from build123d import *

# Parameters (mm, degrees)
F0_R     = 2.5
F0_R_2   = 3.5
F0_W     = 15
F0_H     = 3
F1_DEPTH = 3


with BuildPart() as f1:
    # F0 (on Front) → F1 (new body)
    with BuildSketch(Plane.XZ):
        Polygon((107.5, -32.625), (115, -32.625), (115, 32.625), (107.5, 32.625), (92.5, 32.625), (57.5, 32.625), (42.5, 32.625), (7.5, 32.625), (-7.5, 32.625), (-42.5, 32.625), (-57.5, 32.625), (-92.5, 32.625), (-107.5, 32.625), (-115, 32.625), (-115, -32.625), (-107.5, -32.625), (-92.5, -32.625), (-57.5, -32.625), (-42.5, -32.625), (-7.5, -32.625), (7.5, -32.625), (42.5, -32.625), (57.5, -32.625), (92.5, -32.625), align=None)
        with Locations((-75, -22.375)):
            Circle(F0_R, mode=Mode.SUBTRACT)
        with Locations((-65, -22.375)):
            Circle(F0_R, mode=Mode.SUBTRACT)
        with Locations((-55, -22.375)):
            Circle(F0_R, mode=Mode.SUBTRACT)
        with Locations((-45, -22.375)):
            Circle(F0_R, mode=Mode.SUBTRACT)
        with Locations((-95, -12.375)):
            Circle(F0_R, mode=Mode.SUBTRACT)
        with Locations((-85, -12.375)):
            Circle(F0_R, mode=Mode.SUBTRACT)
        with Locations((-65, -12.375)):
            Circle(F0_R, mode=Mode.SUBTRACT)
        with Locations((-105, -2.375)):
            Circle(F0_R, mode=Mode.SUBTRACT)
        with Locations((-95, -2.375)):
            Circle(F0_R, mode=Mode.SUBTRACT)
        with BuildLine():
            Line((-55.5, -9.875), (-55, -9.875))
            Line((-55, -9.875), (-45, -9.875))
            Line((-45, -9.875), (-35, -9.875))
            Line((-35, -9.875), (-25, -9.875))
            Line((-25, -9.875), (-15, -9.875))
            Line((-15, -9.875), (-5, -9.875))
            Line((-5, -9.875), (-4.5, -9.875))
            ThreePointArc((-4.5, -9.875), (-3.085786, -10.460786), (-2.5, -11.875))
            Line((-2.5, -11.875), (-2.5, -12.375))
            Line((-2.5, -12.375), (-2.5, -12.875))
            ThreePointArc((-2.5, -12.875), (-3.085786, -14.289214), (-4.5, -14.875))
            Line((-4.5, -14.875), (-5, -14.875))
            Line((-5, -14.875), (-15, -14.875))
            Line((-15, -14.875), (-25, -14.875))
            Line((-25, -14.875), (-35, -14.875))
            Line((-35, -14.875), (-45, -14.875))
            Line((-45, -14.875), (-55, -14.875))
            Line((-55, -14.875), (-55.5, -14.875))
            ThreePointArc((-55.5, -14.875), (-56.914214, -14.289214), (-57.5, -12.875))
            Line((-57.5, -12.875), (-57.5, -12.375))
            Line((-57.5, -12.375), (-57.5, -11.875))
            ThreePointArc((-57.5, -11.875), (-56.914214, -10.460786), (-55.5, -9.875))
        make_face(mode=Mode.SUBTRACT)
        with Locations((-55, -2.375)):
            Circle(F0_R, mode=Mode.SUBTRACT)
        with Locations((-45, -2.375)):
            Circle(F0_R, mode=Mode.SUBTRACT)
        with BuildLine():
            Line((-35.5, -19.875), (-35, -19.875))
            Line((-35, -19.875), (-25, -19.875))
            Line((-25, -19.875), (-15, -19.875))
            Line((-15, -19.875), (-5, -19.875))
            Line((-5, -19.875), (5, -19.875))
            Line((5, -19.875), (15, -19.875))
            Line((15, -19.875), (25, -19.875))
            Line((25, -19.875), (35, -19.875))
            Line((35, -19.875), (35.5, -19.875))
            ThreePointArc((35.5, -19.875), (36.914214, -20.460786), (37.5, -21.875))
            Line((37.5, -21.875), (37.5, -22.375))
            Line((37.5, -22.375), (37.5, -22.875))
            ThreePointArc((37.5, -22.875), (36.914214, -24.289214), (35.5, -24.875))
            Line((35.5, -24.875), (35, -24.875))
            Line((35, -24.875), (25, -24.875))
            Line((25, -24.875), (15, -24.875))
            Line((15, -24.875), (5, -24.875))
            Line((5, -24.875), (-5, -24.875))
            Line((-5, -24.875), (-15, -24.875))
            Line((-15, -24.875), (-25, -24.875))
            Line((-25, -24.875), (-35, -24.875))
            Line((-35, -24.875), (-35.5, -24.875))
            ThreePointArc((-35.5, -24.875), (-36.914214, -24.289214), (-37.5, -22.875))
            Line((-37.5, -22.875), (-37.5, -22.375))
            Line((-37.5, -22.375), (-37.5, -21.875))
            ThreePointArc((-37.5, -21.875), (-36.914214, -20.460786), (-35.5, -19.875))
        make_face(mode=Mode.SUBTRACT)
        with Locations((45, -22.375)):
            Circle(F0_R, mode=Mode.SUBTRACT)
        with Locations((55, -22.375)):
            Circle(F0_R, mode=Mode.SUBTRACT)
        with Locations((65, -22.375)):
            Circle(F0_R, mode=Mode.SUBTRACT)
        with Locations((75, -22.375)):
            Circle(F0_R, mode=Mode.SUBTRACT)
        with BuildLine():
            Line((4.5, -9.875), (5, -9.875))
            Line((5, -9.875), (15, -9.875))
            Line((15, -9.875), (25, -9.875))
            Line((25, -9.875), (35, -9.875))
            Line((35, -9.875), (45, -9.875))
            Line((45, -9.875), (55, -9.875))
            Line((55, -9.875), (55.5, -9.875))
            ThreePointArc((55.5, -9.875), (56.914214, -10.460786), (57.5, -11.875))
            Line((57.5, -11.875), (57.5, -12.375))
            Line((57.5, -12.375), (57.5, -12.875))
            ThreePointArc((57.5, -12.875), (56.914214, -14.289214), (55.5, -14.875))
            Line((55.5, -14.875), (55, -14.875))
            Line((55, -14.875), (45, -14.875))
            Line((45, -14.875), (35, -14.875))
            Line((35, -14.875), (25, -14.875))
            Line((25, -14.875), (15, -14.875))
            Line((15, -14.875), (5, -14.875))
            Line((5, -14.875), (4.5, -14.875))
            ThreePointArc((4.5, -14.875), (3.085786, -14.289214), (2.5, -12.875))
            Line((2.5, -12.875), (2.5, -12.375))
            Line((2.5, -12.375), (2.5, -11.875))
            ThreePointArc((2.5, -11.875), (3.085786, -10.460786), (4.5, -9.875))
        make_face(mode=Mode.SUBTRACT)
        with BuildLine():
            ThreePointArc((-35, -4.875), (-37.5, -2.375), (-35, 0.125))
            Line((-35, 0.125), (-25, 0.125))
            Line((-25, 0.125), (-15, 0.125))
            Line((-15, 0.125), (-5, 0.125))
            Line((-5, 0.125), (5, 0.125))
            Line((5, 0.125), (15, 0.125))
            Line((15, 0.125), (25, 0.125))
            Line((25, 0.125), (35, 0.125))
            ThreePointArc((35, 0.125), (36.767767, -0.607233), (37.5, -2.375))
            ThreePointArc((37.5, -2.375), (36.767767, -4.142767), (35, -4.875))
            Line((35, -4.875), (25, -4.875))
            Line((25, -4.875), (15, -4.875))
            Line((15, -4.875), (5, -4.875))
            Line((5, -4.875), (-5, -4.875))
            Line((-5, -4.875), (-15, -4.875))
            Line((-15, -4.875), (-25, -4.875))
            Line((-25, -4.875), (-35, -4.875))
        make_face(mode=Mode.SUBTRACT)
        with Locations((45, -2.375)):
            Circle(F0_R, mode=Mode.SUBTRACT)
        with Locations((55, -2.375)):
            Circle(F0_R, mode=Mode.SUBTRACT)
        with Locations((65, -12.375)):
            Circle(F0_R, mode=Mode.SUBTRACT)
        with Locations((85, -12.375)):
            Circle(F0_R, mode=Mode.SUBTRACT)
        with Locations((95, -12.375)):
            Circle(F0_R, mode=Mode.SUBTRACT)
        with Locations((95, -2.375)):
            Circle(F0_R, mode=Mode.SUBTRACT)
        with Locations((105, -2.375)):
            Circle(F0_R, mode=Mode.SUBTRACT)
        with Locations((-105, 7.625)):
            Circle(F0_R, mode=Mode.SUBTRACT)
        with Locations((-75, 7.625)):
            Circle(F0_R_2, mode=Mode.SUBTRACT)
        with Locations((-45, 7.625)):
            Circle(F0_R, mode=Mode.SUBTRACT)
        with Locations((-35, 7.625)):
            Circle(F0_R, mode=Mode.SUBTRACT)
        with Locations((-25, 7.625)):
            Circle(F0_R, mode=Mode.SUBTRACT)
        with Locations((-15, 7.625)):
            Circle(F0_R, mode=Mode.SUBTRACT)
        with Locations((-5, 7.625)):
            Circle(F0_R, mode=Mode.SUBTRACT)
        with Locations((-5, 17.625)):
            Circle(F0_R, mode=Mode.SUBTRACT)
        with Locations((5, 7.625)):
            Circle(F0_R, mode=Mode.SUBTRACT)
        with Locations((15, 7.625)):
            Circle(F0_R, mode=Mode.SUBTRACT)
        with Locations((25, 7.625)):
            Circle(F0_R, mode=Mode.SUBTRACT)
        with Locations((35, 7.625)):
            Circle(F0_R, mode=Mode.SUBTRACT)
        with Locations((45, 7.625)):
            Circle(F0_R, mode=Mode.SUBTRACT)
        with Locations((5, 17.625)):
            Circle(F0_R, mode=Mode.SUBTRACT)
        with Locations((75, 7.625)):
            Circle(F0_R_2, mode=Mode.SUBTRACT)
        with Locations((105, 7.625)):
            Circle(F0_R, mode=Mode.SUBTRACT)
        with Locations((100, -34.125)):
            Rectangle(F0_W, F0_H)
        with Locations((100, 34.125)):
            Rectangle(F0_W, F0_H)
        with Locations((50, -34.125)):
            Rectangle(F0_W, F0_H)
        with Locations((50, 34.125)):
            Rectangle(F0_W, F0_H)
        with Locations((0, -34.125)):
            Rectangle(F0_W, F0_H)
        with Locations((0, 34.125)):
            Rectangle(F0_W, F0_H)
        with Locations((-50, -34.125)):
            Rectangle(F0_W, F0_H)
        with Locations((-50, 34.125)):
            Rectangle(F0_W, F0_H)
        with Locations((-100, -34.125)):
            Rectangle(F0_W, F0_H)
        with Locations((-100, 34.125)):
            Rectangle(F0_W, F0_H)
    extrude(amount=F1_DEPTH)


solid = f1.part
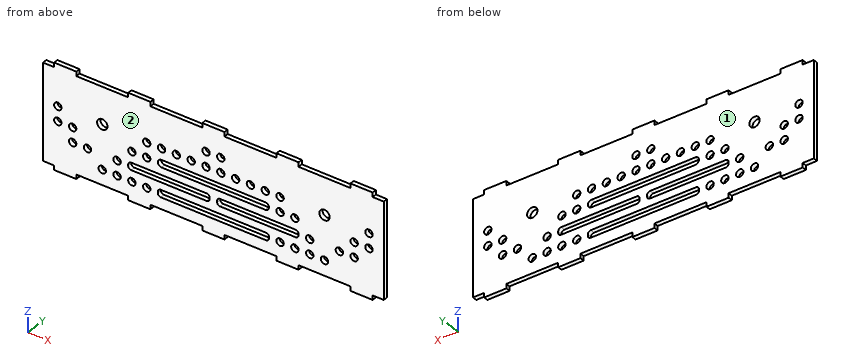
Geometry: final body of the model. Coordinates: model frame, mm. Face numbers are marked on the shaded views. Round coordinates to 2 decimals unless told otherwise and drop trailing zeros. Order: outer loops, then holes, each group sorted by start corner. A loop starts at its lowest first (then second) coordinate and runs counter-clockwise, first axis right, second up. Notation, with made-up numbers: (86.25, 54) -> (116.25, 54) arc R20 cw to (116.25, 76) -> close; hole circle Ø9 at (71.25, -34). An arc over 180 degrees is marked (long way). Put each result on its own line as item: value. Start each with the question number.
Q1. Pull-direction query (Y, two-part tool) for the marked faces 1 and 2; classes: +Y half, -Y half, draft (parallel to the pull), parting line (faces both ways), or undercut.
Q2. Section A-A on x = 25. Return the cut outline in (y, z) (3 decimals).
Q3. Section D-D on y = -1.8. Give the number of separate pieces and of enclosed holes in the cut face, and give its area (3 significant figures).
Q4. Section C-C on x = -95. Return the cut outline in (y, z) (3 decimals), and give its area (3 significant figures).
Q5. Section B-B on x = -65. Return the cut outline in (y, z) (3 decimals).
Q6. First-contact query: pin 1 (1.5 mm diameter, centred on x = -40, y = -2, fed in from -Z) (3 decimals); pin 2 (3 mm diameter, centred on x = -5, z = 7.625, fed in from +Y); pin 3 (1.5 mm diameter, centred on y = -2, z = -34.5, fed in from +X); pin 4 (8 mm diameter, centred on x = 105, z = 7.625, fed in from -Y). Flat tips, straight axial feed; report the tip coordinate or a pass-through.
Q7. Line query: probe 1 along Z at (x, y) = (9, -0.7) (3 decimals); probe 2 along Z at (x, y) = (-95, -1.7) (3 decimals); probe 3 along Z at (x, y) = (4, -2.55) (1 decimal). Output: solid intervals per line, ascending.
Ans:
1. face 1: +Y half
1. face 2: -Y half
2. outline: (-3, -32.625) -> (0, -32.625) -> (0, -24.875) -> (-3, -24.875) -> close; (-3, -19.875) -> (0, -19.875) -> (0, -14.875) -> (-3, -14.875) -> close; (-3, -9.875) -> (0, -9.875) -> (0, -4.875) -> (-3, -4.875) -> close; (-3, 0.125) -> (0, 0.125) -> (0, 5.125) -> (-3, 5.125) -> close; (-3, 10.125) -> (0, 10.125) -> (0, 32.625) -> (-3, 32.625) -> close
3. separate pieces: 1
3. enclosed holes: 42
3. area: 13,400 mm2
4. outline: (-3, -35.625) -> (0, -35.625) -> (0, -14.875) -> (-3, -14.875) -> close; (-3, -9.875) -> (0, -9.875) -> (0, -4.875) -> (-3, -4.875) -> close; (-3, 0.125) -> (0, 0.125) -> (0, 35.625) -> (-3, 35.625) -> close
4. area: 184 mm2
5. outline: (-3, -32.625) -> (0, -32.625) -> (0, -24.875) -> (-3, -24.875) -> close; (-3, -19.875) -> (0, -19.875) -> (0, -14.875) -> (-3, -14.875) -> close; (-3, -9.875) -> (0, -9.875) -> (0, 32.625) -> (-3, 32.625) -> close
6. pin 1: stops at z = -32.625
6. pin 2: passes through
6. pin 3: stops at x = 107.5
6. pin 4: stops at y = -3
7. probe 1: z = -32.625 to -24.875, -19.875 to -14.875, -9.875 to -4.875, 0.125 to 32.625
7. probe 2: z = -35.625 to -14.875, -9.875 to -4.875, 0.125 to 35.625
7. probe 3: z = -35.6 to -24.9, -19.9 to -14.8, -9.9 to -4.9, 0.1 to 5.3, 9.9 to 15.3, 19.9 to 35.6
